Solid Edge part; units mm, degrees
sketch "Sketch1" plane through (0, 0, 0) normal (0, 0, 1) x (1, 0, 0)
  line L0 (-19.75, -8.15) -> (19.75, -8.15)
  line L1 (19.75, -8.15) -> (19.75, 8.15)
  line L2 (19.75, 8.15) -> (-19.75, 8.15)
  line L3 (-19.75, 8.15) -> (-19.75, -8.15)
  dimension "D1" = 19.75
  dimension "D2" = 19.75
extrude "Protrusion1" add sketch "Sketch1" along normal blind 1.25
sketch "Sketch2" plane through (0, 0, 1.25) normal (0, 0, 1) x (1, 0, 0)
  line L0 (13.5, 8.15) -> (0.7, 8.15)
  line L1 (0.7, 8.15) -> (0.7, 1.55)
  line L2 (0.7, 1.55) -> (13.5, 1.55)
  line L3 (13.5, 1.55) -> (13.5, 8.15)
  dimension "D1" = 13.5
  dimension "D2" = 13.5
extrude "ExtrudedProtrusion_2" add sketch "Sketch2" along normal blind 5.8
sketch "Sketch3" plane through (0, 0, 1.25) normal (0, 0, 1) x (1, 0, 0)
  line L0 (-16.15, 6.55) -> (-8.85, 6.55)
  line L1 (-8.85, 6.55) -> (-8.85, -5.95)
  line L2 (-8.85, -5.95) -> (-16.15, -5.95)
  line L3 (-16.15, -5.95) -> (-16.15, 6.55)
  dimension "D1" = 16.15
  dimension "D2" = 8.85
extrude "ExtrudedProtrusion_3" add sketch "Sketch3" along normal blind 6
hole "Hole_1" at (16.55, 5.15, 1.25) direction (0, 0, -1) diameter 3.5 end up to next
hole "Hole1" at (-2.45, 5.15, 1.25) direction (0, 0, -1) diameter 3.5 end up to next
sketch "Sketch4" plane through (7.1, 4.85, 7.05) normal (0, 0, 1) x (1, 0, 0)
  line L0 (-5.4, 3.3) -> (7.1, 8.3)
  line L1 (7.1, 8.3) -> (7.1, 7.7615)
  line L2 (7.1, 7.7615) -> (-4.0537, 3.3)
  line L3 (-4.0537, 3.3) -> (-5.4, 3.3)
extrude "ExtrudedProtrusion_4" add sketch "Sketch4" against normal blind 4.8
sketch "Sketch5" plane through (0.7, 4.85, 4.15) normal (-1, 0, 0) x (0, -1, 0)
  line L0 (-3.3, 2.9) -> (-3.3, 1.9)
  line L1 (-3.3, 1.9) -> (-8.3, 1.9)
  line L2 (-8.3, 1.9) -> (-8.3, 2.9)
  line L3 (-8.3, 2.9) -> (-3.3, 2.9)
  dimension "D1" = 3.3
extrude "Cutout1" cut sketch "Sketch5" against normal up to next
properties material "Polyethylene, low density"
CAD build for the part. Positions are in the model's coordinates, mm. A direction names the side the tool comes from. Round coordinates to 2 decimals unless told otherwise and drop trailing zeros. Loops run counter-clockwise (first coordinate to the right, second up) from the corner with the lowest first, then second, coordinate; pieces in that order, holes last. Notation, with made-up numbers: (13, -14.75) - (71, -14.75) arc R28 cw to (71, 13.25) - close; hole circle Ø4 at (14, 61). An arc over 180 degrees is marked (long way). Put each result on its own line as item: value.
1. Pin check, flat tips, straight feed: P1, Ø4, axis at x = 16.55, y = 5.15, coming from the +Z side; P2, Ø3, axis at x = 6.5, z = 3, coming from the -Y side; P3, Ø1.5, axis at x = 10.5, y = 10.5, coming from the -Z side. Stop position of each tip, or through.
Geometry check:
P1: z = 1.25
P2: y = 1.55
P3: z = 2.25
2. Slice it at D-D on x = -15.5. List the corners of the cut face in (y, z), and give its area (3 significant figures).
Geometry check:
outline: (-8.15, 0) - (8.15, 0) - (8.15, 1.25) - (6.55, 1.25) - (6.55, 7.25) - (-5.95, 7.25) - (-5.95, 1.25) - (-8.15, 1.25) - close
area: 95.4 mm²
3. 3-axis set-ups, long thin cutter, end or side, ignore diameter. For faces 1 (the flat face through (-12, -5.95, 4)), 2 (the flat face through (0.7, 5, 4)), 3 (the flat face through (13.5, 5, 4)), 4 (the flat face through (7, 5, 7.05)): which of +Z, -Z, +X, -X, +Y, -Y reach the whole face in a straight line?
Geometry check:
face 1: +Z, +X, -X, -Y
face 2: +Z, +Y, -Y
face 3: +Z, +X, -Y
face 4: +Z, +X, +Y, -Y
4. Slice it at B-B on x = -2.45. List the corners of the cut face in (y, z), and give its area (3 significant figures).
Geometry check:
outline: (-8.15, 0) - (3.4, 0) - (3.4, 1.25) - (-8.15, 1.25) - close; (6.9, 0) - (8.15, 0) - (8.15, 1.25) - (6.9, 1.25) - close
area: 16.0 mm²
5. Slice it at A-A on z = 1.75. List the corners of the cut face in (x, y).
Geometry check:
outline: (-16.15, -5.95) - (-8.85, -5.95) - (-8.85, 6.55) - (-16.15, 6.55) - close; (0.7, 1.55) - (13.5, 1.55) - (13.5, 8.15) - (0.7, 8.15) - close
6. Two-plate mould, pull along X, no slides. Class faces 5 (the flat face through (-8.85, 0, 4)), 6 (the flat face through (7.863, 10.615, 4.177)), 7 (the flat face through (8.4, 10.5, 2.25)): released by +X, released by -X, zero draft, split by the parting line, or undercut.
Geometry check:
face 5: undercut
face 6: released by -X
face 7: zero draft
7. Slice it at C-C on y = 5.15. List the corners of the cut face in (x, z).
Geometry check:
outline: (-19.75, 0) - (-4.2, 0) - (-4.2, 1.25) - (-8.85, 1.25) - (-8.85, 7.25) - (-16.15, 7.25) - (-16.15, 1.25) - (-19.75, 1.25) - close; (-0.7, 0) - (14.8, 0) - (14.8, 1.25) - (13.5, 1.25) - (13.5, 7.05) - (0.7, 7.05) - (0.7, 1.25) - (-0.7, 1.25) - close; (18.3, 0) - (19.75, 0) - (19.75, 1.25) - (18.3, 1.25) - close
8. Wall check: line 1 (X direction, y = 5.15, z = 0.65); line 2 (Y direction, x = 16.55, z = 0.5); line 3 (Z direction, x = 0.5, y = -0.75). Give the ranges that are in metal, low to high.
Geometry check:
line 1: -19.75 to -4.2, -0.7 to 14.8, 18.3 to 19.75
line 2: -8.15 to 3.4, 6.9 to 8.15
line 3: 0 to 1.25
